Input: part model. Units: mm. Frame: model coordinates. A direction names the side the tool comes from. Give positions to 0.01 mm unless a question says otherwise; leave off trailing zeros. Write each loop counter-clockwise with the first axis right and the second up, starting at its lowest first coordinate (ties: lowest second). Pieces come first, ordered by that corner, then holes.
```python
from build123d import *

# Parameters (mm, degrees)
F0_R     = 3.25
F1_DEPTH = 1.1
F2_R     = 5.1
F3_DEPTH = 8.5
F4_R     = 2.5
F4_R_2   = 1.6
F5_DEPTH = 2
F6_R     = 2.5
F7_DEPTH = 8.5
F8_R     = 0.1
F9_R     = 1.7


with BuildPart() as f1:
    # F0 (on Top) → F1 (new body)
    with BuildSketch(Plane.XY):
        Circle(F0_R)
    extrude(amount=F1_DEPTH)

    # F2 (on face) → F3 (join)
    with BuildSketch(Plane.XY.offset(1.1)):
        Circle(F2_R)
    extrude(amount=F3_DEPTH)

    # F4 (on face) → F5 (join)
    with BuildSketch(Plane.XY.offset(9.6)):
        Circle(F4_R)
        Circle(F4_R_2, mode=Mode.SUBTRACT)
    extrude(amount=F5_DEPTH)

    # F6 (on face) → F7 (cut)
    with BuildSketch(Plane(origin=(0, 0, 0), x_dir=(1, 0, 0), z_dir=(0, 0, -1))):
        Circle(F6_R)
    extrude(amount=-F7_DEPTH, mode=Mode.SUBTRACT)

    # F8
    f8_edges = [f1.edges().sort_by_distance(p)[0] for p in [
        (-3.25, 0, 0),
        (-2.5, 0, 11.6),
        (-1.6, 0, 11.6),
    ]]
    fillet(f8_edges, radius=F8_R)

    # F9
    f9_edges = [f1.edges().sort_by_distance(p)[0] for p in [
        (-5.1, 0, 9.6),
        (-5.1, 0, 1.1),
    ]]
    fillet(f9_edges, radius=F9_R)


solid = f1.part
```
Item 1: Set-up query: faces 4 (the cylindrical face through (-0.54, 2.44, 4.19)), 5 (the flat face through (-2, 2, 0)), 6 (the flat face through (0, 0, 9.6)). Return all of +Z, -Z, +X, -X, +Y, -Y with unobstructed straight access to the full face (end or side cutting, diameter ignored); none if empty.
Item 2: Section D-D (z = 9.75). Return loops of the section in (x, y), and give its area (3 significant figures).
Item 3: Ray query, line 1 (Y direction, x = 0, z = 10.65); line 2 (Y direction, x = 0, z = 3.25); line 3 (X direction, y = 0.75, z = 3). Return the intervals inside material, ascending.
Item 4: Pin query (flat end, axial travel): pin 1 (2 mm diameter, centred on x = 3, y = -1, fed in from +Z); pin 2 (2.5 mm diameter, centred on x = -0.5, y = -1, fed in from -Z); pin 3 (1 mm diameter, centred on y = -2, z = 2, fed in from -X); pin 4 (1.6 mm diameter, centred on x = 0, y = 0, fed in from +Z). Return the tip coordinate at first contact, or that it passes through.
Item 5: Mould query, pull axis X, two halves, no side actions, for faces 1 (the cylindrical face through (2.4, -4.5, 5.3)), 2 (the cylindrical face through (-1.27, -0.97, 10.54)), 3 (the flat face through (-2, 2, 9.6)). Classes: +X half, -X half, draft (parallel to the pull), parting line (faces both ways), or undercut.
Item 6: Section C-C (z = 7.75). Return loops of the section in (x, y), and give its area (3 significant figures).
Solved:
1. face 4: -Z
1. face 5: -Z, +X, -X, +Y, -Y
1. face 6: +Z
2. outline: circle Ø5 at (0, 0); hole circle Ø3.2 at (0, 0)
2. area: 11.6 mm2
3. line 1: y = -2.5 to -1.6, 1.6 to 2.5
3. line 2: y = -5.1 to -2.5, 2.5 to 5.1
3. line 3: x = -5.04 to -2.38, 2.38 to 5.04
4. pin 1: stops at z = 11.6
4. pin 2: stops at z = 8.5
4. pin 3: stops at x = -4.76
4. pin 4: stops at z = 9.6
5. face 1: parting line
5. face 2: undercut
5. face 3: draft
6. outline: circle Ø10.2 at (0, 0); hole circle Ø5 at (0, 0)
6. area: 62.1 mm2
